The figure shows three views and two pictorial views of one solid part (mm, origin at its lowest corner). Answer the questions. Round coordinates to 2 decimals unless told otherwise and drop trailing zeros. Order: outer loops, then holes, each group sorted by start corner. A loop starts at its lowest first (then second) coordinate and runs counter-clockwise, first axis right, second up. Notation, with made-up numbers: M -6,21 L 13,21 A16 ccw 13,25 Z; hole C 86.5,65.25 d8. An arc over 180 degrees is marked long. Answer as CSV lines item,"result".
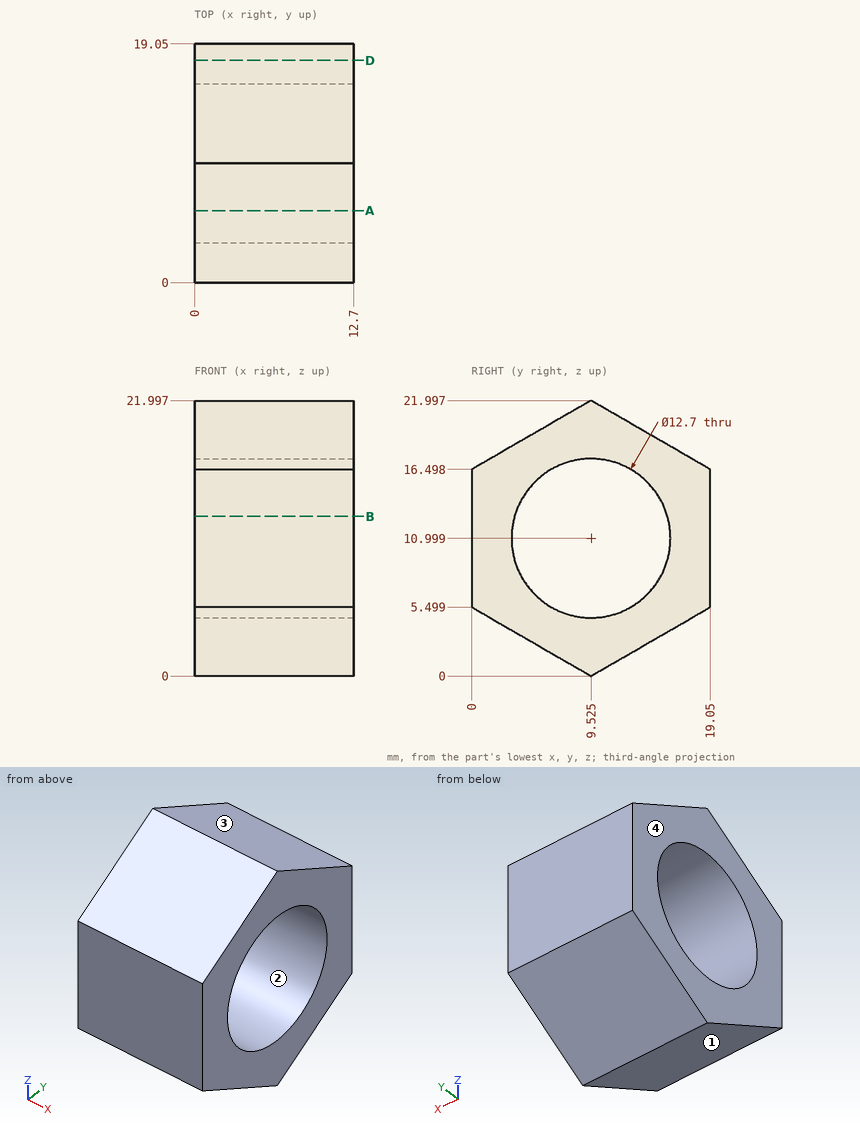
Item 1: Find the intervals of material crossed by probe 1 along Y at (x, z) = (1, 13.25); probe 2 along Y at (x, z) = (9, 6.25); probe 3 along Z at (x, y) = (2.25, 9.75) (1 decimal), in increasing order. Write a range as [from, to].
Ans:
probe 1,"[0, 3.59], [15.46, 19.05]"
probe 2,"[0, 5.31], [13.74, 19.05]"
probe 3,"[0.1, 4.7], [17.3, 21.9]"
Item 2: Determine the mould class of the marked faces 1, 2, 3 and 4 for opening direction Z: +Z half, -Z half, draft (parallel to the pull), parting line (faces both ways), or undercut.
Ans:
face 1,"-Z half"
face 2,"undercut"
face 3,"+Z half"
face 4,"draft"
Item 3: A cutting plane is placed at B-B, the plane z = 12.75. Determine the outline of the cut face in (x, y).
Ans:
outline,"M 0,0 L 12.7,0 L 12.7,3.42 L 0,3.42 Z; M 0,15.63 L 12.7,15.63 L 12.7,19.05 L 0,19.05 Z"
Item 4: Flat-ended cylindrical pins translate along their axes: pin 1 (2 mm diameter, centred on x = 2.5, z = 2.5, fed in from -Y) (1 decimal); pin 2 (6 mm diameter, centred on x = 1.5, z = 18.5, fed in from +Y). Find the tip coordinate at first contact, or state that the pin passes through.
Ans:
pin 1,"y = 3.5"
pin 2,"y = 19.05"
Item 5: A cutting plane is placed at A-A, the plane y = 5.75. Determine the outline of the cut face in (x, z) (1 decimal).
Ans:
outline,"M 0,2.2 L 12.7,2.2 L 12.7,5.9 L 0,5.9 Z; M 0,16.1 L 12.7,16.1 L 12.7,19.8 L 0,19.8 Z"
Item 6: A cutting plane is placed at D-D, the plane y = 17.75. Determine the outline of the cut face in (x, z), and give its area (3 significant figures).
Ans:
outline,"M 0,4.75 L 12.7,4.75 L 12.7,17.25 L 0,17.25 Z"
area,"159 mm2"
